Verification items for the finished model (mm, model axes). A direction names the side the tool comes from. Round coordinates to 2 decimals unless told otherwise and drop trailing zeros. Write each loop counter-clockwise with the first axis right and the second up, starting at its lowest first coordinate (ties: lowest second). Pieces come first, ordered by that corner, then holes. Notation, with made-up numbers: (47.5, 52) - (102.5, 52) arc R6 cw to (102.5, 58) - close; hole circle Ø4 at (-32.5, 55.25). An arc over 180 degrees is marked (long way). Answer as a JSON object with one key per item and string values. Group by question number.
1) Go/stop test with flat-tipped pins: pin 1 Ø1 at (x, z) = (42, -46.5) entering from -Y; pin 2 Ø12 at (y, z) = (37, -9.5) entering from +X; pin 3 Ø6 at (x, z) = (-20, -58) entering from +Y; pin 4 Ø9 at (x, y) = (0, 0) entering from -Z. Record where each tip stops, or that it passes through.
2) Section check B-B (z = 2). Enter the section's corners in (x, y), then the cut area to 3 significant figures.
3) Mould release check, pull along X, two halves, no side actions. Record for faces 1 (the flat face through (0, -40, -35)), 2 (the flat face through (22, 40, 0)), 3 (the flat face through (13, -4, 0)): +X half, -X half, draft (parallel to the pull), parting line (faces both ways), or undercut.
4) Section check A-A (z = -25.5). Enter the section's corners in (x, y).
5) Thickness scan on line 1 (Y direction, x = 12, z = -5.5); line 2 (Y direction, x = 0, z = 4.75); line 3 (Y direction, x = 45.5, z = -59.5). Record the ranges inside material, lowest first.
6) Section check D-D (x = -37). Enter the section's corners in (y, z).
7) Section check C-C (y = -2.5). Enter the section's corners in (x, z).
8) Set-up check for faces 4 (the flat face through (34, -20, -35)), 5 (the flat face through (-34.186, -19.225, -34.51)), 6 (the flat face through (-10.828, 6.307, -34.51)): record each of +Z, -Z, +X, -X, +Y, -Y from which the full face is reachable in a straight line by a thin tool's end or side.
```python
from build123d import *

# Parameters (mm, degrees)
F0_R     = 5
F1_DEPTH = 7
F2_DEPTH = 70


# Not quite as in the source:
# - after a boolean that leaves OpenCascade's solid faulty, fix() repairs it


with BuildPart() as f1:
    # F0 (on Top) → F1 (new body)
    with BuildSketch(Plane.XY):
        with BuildLine():
            Line((11.5470053838, 20), (56.5685424949, 20))
            ThreePointArc((56.5685424949, 20), (30, 51.9615242271), (-10.9637631718, 58.9897948557))
            Line((-10.9637631718, 58.9897948557), (11.5470053838, 20))
        make_face()
        with BuildLine():
            ThreePointArc((-10.9637631718, -58.9897948557), (30, -51.9615242271), (56.5685424949, -20))
            Line((56.5685424949, -20), (11.5470053838, -20))
            Line((11.5470053838, -20), (-10.9637631718, -58.9897948557))
        make_face()
        with BuildLine():
            ThreePointArc((58.5747385824, -13), (59.6426203103, -6.5389481208), (60, 0))
            ThreePointArc((60, 0), (59.6426203103, 6.5389481208), (58.5747385824, 13))
            Line((58.5747385824, 13), (15.5884572681, 13))
            Line((15.5884572681, 13), (7.5055534995, 13))
            Line((7.5055534995, 13), (11.2583302492, 6.5))
            ThreePointArc((11.2583302492, 6.5), (12.5570357418, 3.3646475863), (13, 0))
            ThreePointArc((13, 0), (12.5570357418, -3.3646475863), (11.2583302492, -6.5))
            Line((11.2583302492, -6.5), (7.5055534995, -13))
            Line((7.5055534995, -13), (15.5884572681, -13))
            Line((15.5884572681, -13), (58.5747385824, -13))
        make_face()
        with BuildLine():
            ThreePointArc((56.5685424949, -20), (57.6779316057, -16.5304629604), (58.5747385824, -13))
            Line((58.5747385824, -13), (15.5884572681, -13))
            Line((15.5884572681, -13), (11.5470053838, -20))
            Line((11.5470053838, -20), (56.5685424949, -20))
        make_face()
        with BuildLine():
            Line((15.5884572681, 13), (58.5747385824, 13))
            ThreePointArc((58.5747385824, 13), (57.6779316057, 16.5304629604), (56.5685424949, 20))
            Line((56.5685424949, 20), (11.5470053838, 20))
            Line((11.5470053838, 20), (15.5884572681, 13))
        make_face()
        with BuildLine():
            Line((3.4641016151, -20), (7.5055534995, -13))
            Line((7.5055534995, -13), (0, -13))
            ThreePointArc((0, -13), (-6.6785653008, -11.1533297953), (-11.4597294399, -6.1379639265))
            Line((-11.4597294399, -6.1379639265), (-14.736550409, -0.4623435209))
            Line((-14.736550409, -0.4623435209), (-18.7780022933, -7.4623435209))
            Line((-18.7780022933, -7.4623435209), (-40.1906368837, -44.5501145553))
            ThreePointArc((-40.1906368837, -44.5501145553), (-29.7919429343, -52.081091926), (-18.029039042, -57.2272116324))
            Line((-18.029039042, -57.2272116324), (3.4641016151, -20))
        make_face()
        with BuildLine():
            Line((-14.736550409, -0.4623435209), (-40.5407150531, 44.2317806897))
            ThreePointArc((-40.5407150531, 44.2317806897), (-43.1499853268, 41.6902718424), (-45.6002292233, 38.995116294))
            Line((-45.6002292233, 38.995116294), (-23.0863883339, 0))
            Line((-23.0863883339, 0), (-18.7780022933, -7.4623435209))
            Line((-18.7780022933, -7.4623435209), (-14.736550409, -0.4623435209))
        make_face()
        with BuildLine():
            Line((0, 13), (7.5055534995, 13))
            Line((7.5055534995, 13), (3.4641016151, 20))
            Line((3.4641016151, 20), (-18.029039042, 57.2272116324))
            ThreePointArc((-18.029039042, 57.2272116324), (-29.9970720244, 51.9632145846), (-40.5407150531, 44.2317806897))
            Line((-40.5407150531, 44.2317806897), (-14.736550409, -0.4623435209))
            Line((-14.736550409, -0.4623435209), (-12.5822883529, 3.2689478131))
            ThreePointArc((-12.5822883529, 3.2689478131), (-11.2583302492, 6.5), (-9.1221360262, 9.2621074448))
            ThreePointArc((-9.1221360262, 9.2621074448), (-4.9291278751, 12.0292850324), (0, 13))
        make_face()
        with BuildLine():
            Line((-23.0863883339, 0), (-45.6002292233, 38.995116294))
            ThreePointArc((-45.6002292233, 38.995116294), (-60, 0), (-45.6002292233, -38.995116294))
            Line((-45.6002292233, -38.995116294), (-23.0863883339, 0))
        make_face()
        with BuildLine():
            Line((11.5470053838, 20), (-10.9637631718, 58.9897948557))
            ThreePointArc((-10.9637631718, 58.9897948557), (-14.5231649428, 58.2157854885), (-18.029039042, 57.2272116324))
            Line((-18.029039042, 57.2272116324), (3.4641016151, 20))
            Line((3.4641016151, 20), (11.5470053838, 20))
        make_face()
        with BuildLine():
            ThreePointArc((-45.6002292233, -38.995116294), (-42.9852611748, -41.8600922328), (-40.1906368837, -44.5501145553))
            Line((-40.1906368837, -44.5501145553), (-18.7780022933, -7.4623435209))
            Line((-18.7780022933, -7.4623435209), (-23.0863883339, 0))
            Line((-23.0863883339, 0), (-45.6002292233, -38.995116294))
        make_face()
        with BuildLine():
            ThreePointArc((-18.029039042, -57.2272116324), (-14.5231649428, -58.2157854885), (-10.9637631718, -58.9897948557))
            Line((-10.9637631718, -58.9897948557), (11.5470053838, -20))
            Line((11.5470053838, -20), (3.4641016151, -20))
            Line((3.4641016151, -20), (-18.029039042, -57.2272116324))
        make_face()
        Polygon((11.5470053838, -20), (15.5884572681, -13), (7.5055534995, -13), (3.4641016151, -20), align=None)
        Polygon((7.5055534995, 13), (15.5884572681, 13), (11.5470053838, 20), (3.4641016151, 20), align=None)
        with BuildLine():
            Line((0, -13), (7.5055534995, -13))
            Line((7.5055534995, -13), (11.2583302492, -6.5))
            ThreePointArc((11.2583302492, -6.5), (6.5, -11.2583302492), (0, -13))
        make_face()
        with BuildLine():
            Line((-12.5822883529, 3.2689478131), (-9.1221360262, 9.2621074448))
            ThreePointArc((-9.1221360262, 9.2621074448), (-11.2583302492, 6.5), (-12.5822883529, 3.2689478131))
        make_face()
        with BuildLine():
            Line((11.2583302492, 6.5), (7.5055534995, 13))
            Line((7.5055534995, 13), (0, 13))
            ThreePointArc((0, 13), (6.5, 11.2583302492), (11.2583302492, 6.5))
        make_face()
        with BuildLine():
            Line((-14.736550409, -0.4623435209), (-11.4597294399, -6.1379639265))
            ThreePointArc((-11.4597294399, -6.1379639265), (-12.9084140005, -1.5404051392), (-12.5822883529, 3.2689478131))
            Line((-12.5822883529, 3.2689478131), (-14.736550409, -0.4623435209))
        make_face()
        with BuildLine():
            ThreePointArc((11.2583302492, 6.5), (6.5, 11.2583302492), (0, 13))
            ThreePointArc((0, 13), (-4.9291278751, 12.0292850324), (-9.1221360262, 9.2621074448))
            Line((-9.1221360262, 9.2621074448), (-12.5822883529, 3.2689478131))
            ThreePointArc((-12.5822883529, 3.2689478131), (-12.9084140005, -1.5404051392), (-11.4597294399, -6.1379639265))
            ThreePointArc((-11.4597294399, -6.1379639265), (-6.6785653008, -11.1533297953), (0, -13))
            ThreePointArc((0, -13), (6.5, -11.2583302492), (11.2583302492, -6.5))
            ThreePointArc((11.2583302492, -6.5), (12.5570357418, -3.3646475863), (13, 0))
            ThreePointArc((13, 0), (12.5570357418, 3.3646475863), (11.2583302492, 6.5))
        make_face()
        Circle(F0_R, mode=Mode.SUBTRACT)
    extrude(amount=F1_DEPTH)

    # F0 (on Top) → F2 (join)
    with BuildSketch(Plane.XY):
        with BuildLine():
            ThreePointArc((56.5685424949, -20), (57.6779316057, -16.5304629604), (58.5747385824, -13))
            Line((58.5747385824, -13), (15.5884572681, -13))
            Line((15.5884572681, -13), (11.5470053838, -20))
            Line((11.5470053838, -20), (56.5685424949, -20))
        make_face()
        Polygon((11.5470053838, -20), (15.5884572681, -13), (7.5055534995, -13), (3.4641016151, -20), align=None)
        with BuildLine():
            ThreePointArc((-18.029039042, -57.2272116324), (-14.5231649428, -58.2157854885), (-10.9637631718, -58.9897948557))
            Line((-10.9637631718, -58.9897948557), (11.5470053838, -20))
            Line((11.5470053838, -20), (3.4641016151, -20))
            Line((3.4641016151, -20), (-18.029039042, -57.2272116324))
        make_face()
        with BuildLine():
            ThreePointArc((-45.6002292233, -38.995116294), (-42.9852611748, -41.8600922328), (-40.1906368837, -44.5501145553))
            Line((-40.1906368837, -44.5501145553), (-18.7780022933, -7.4623435209))
            Line((-18.7780022933, -7.4623435209), (-23.0863883339, 0))
            Line((-23.0863883339, 0), (-45.6002292233, -38.995116294))
        make_face()
        with BuildLine():
            Line((-14.736550409, -0.4623435209), (-40.5407150531, 44.2317806897))
            ThreePointArc((-40.5407150531, 44.2317806897), (-43.1499853268, 41.6902718424), (-45.6002292233, 38.995116294))
            Line((-45.6002292233, 38.995116294), (-23.0863883339, 0))
            Line((-23.0863883339, 0), (-18.7780022933, -7.4623435209))
            Line((-18.7780022933, -7.4623435209), (-14.736550409, -0.4623435209))
        make_face()
        with BuildLine():
            Line((11.5470053838, 20), (-10.9637631718, 58.9897948557))
            ThreePointArc((-10.9637631718, 58.9897948557), (-14.5231649428, 58.2157854885), (-18.029039042, 57.2272116324))
            Line((-18.029039042, 57.2272116324), (3.4641016151, 20))
            Line((3.4641016151, 20), (11.5470053838, 20))
        make_face()
        Polygon((7.5055534995, 13), (15.5884572681, 13), (11.5470053838, 20), (3.4641016151, 20), align=None)
        with BuildLine():
            Line((15.5884572681, 13), (58.5747385824, 13))
            ThreePointArc((58.5747385824, 13), (57.6779316057, 16.5304629604), (56.5685424949, 20))
            Line((56.5685424949, 20), (11.5470053838, 20))
            Line((11.5470053838, 20), (15.5884572681, 13))
        make_face()
        with BuildLine():
            ThreePointArc((11.2583302492, 6.5), (6.5, 11.2583302492), (0, 13))
            ThreePointArc((0, 13), (-4.9291278751, 12.0292850324), (-9.1221360262, 9.2621074448))
            Line((-9.1221360262, 9.2621074448), (-12.5822883529, 3.2689478131))
            ThreePointArc((-12.5822883529, 3.2689478131), (-12.9084140005, -1.5404051392), (-11.4597294399, -6.1379639265))
            ThreePointArc((-11.4597294399, -6.1379639265), (-6.6785653008, -11.1533297953), (0, -13))
            ThreePointArc((0, -13), (6.5, -11.2583302492), (11.2583302492, -6.5))
            ThreePointArc((11.2583302492, -6.5), (12.5570357418, -3.3646475863), (13, 0))
            ThreePointArc((13, 0), (12.5570357418, 3.3646475863), (11.2583302492, 6.5))
        make_face()
        Circle(F0_R, mode=Mode.SUBTRACT)
    extrude(amount=-F2_DEPTH)

    add(f1.part.fix(), mode=Mode.REPLACE)


solid = f1.part
```
Returned:
{
 "1": {"pin 1": "y = -20", "pin 2": "x = 5.2", "pin 3": "y = 57.54", "pin 4": "through"},
 "2": {"outline": "circle Ø120 at (0, 0); hole circle Ø10 at (0, 0)", "area": "11,200 mm2"},
 "3": {"face 1": "+X half", "face 2": "draft", "face 3": "undercut"},
 "4": {"outline": "(-45.6, -39) arc R60 ccw to (-40.19, -44.55) - (-14.74, -0.46) - (-40.54, 44.23) arc R60 ccw to (-45.6, 39) - (-23.09, 0) - close; (-18.03, -57.23) arc R60 ccw to (-10.96, -58.99) - (11.55, -20) - (56.57, -20) arc R60 ccw to (58.57, -13) - (7.51, -13) - close; (-18.03, 57.23) - (7.51, 13) - (58.57, 13) arc R60 ccw to (56.57, 20) - (11.55, 20) - (-10.96, 58.99) arc R60 ccw to start; (-12.58, 3.27) arc R13 ccw (long way) to (-9.12, 9.26) - close; hole circle Ø10 at (0, 0)"},
 "5": {"line 1": "-20 to -13, -5 to 5, 13 to 20", "line 2": "-60 to -5, 5 to 60", "line 3": "-20 to -13, 13 to 20"},
 "6": {"outline": "(-47.23, 0) - (-39.02, 0) - (-39.02, -70) - (-24.1, -70) - (-24.1, 0) - (24.1, 0) - (24.1, -70) - (38.1, -70) - (38.1, 0) - (47.23, 0) - (47.23, 7) - (-47.23, 7) - close"},
 "7": {"outline": "(-59.95, 0) - (-24.53, 0) - (-24.53, -70) - (-15.91, -70) - (-15.91, 0) - (-12.76, 0) - (-12.76, -70) - (-4.33, -70) - (-4.33, 7) - (-59.95, 7) - close; (4.33, -70) - (12.76, -70) - (12.76, 0) - (59.95, 0) - (59.95, 7) - (4.33, 7) - close"},
 "8": {"face 4": "-Z, +X, -Y", "face 5": "-Z, -X", "face 6": "-Z"}
}
